Answer from the drawing. Dimensions are ordinates in mm from the lowest x, y and z of the part. A direction names the side the tool comes from. Give positions to 0.01 mm unless a question says otherwise; leave off trailing zeros. Loops run counter-clockwise (first coordinate to the right, second up) from the corner with the lowest first, then second, coordinate; pieces in that order, holes last.
Item 1: Consider line 1 along X through (y, z) = (3.35, 15.5); line 2 along Y through (x, z) = (4, 23.15); line 3 along X through (y, z) = (2.3, 5.5). Determine where each line is inside the solid, lowest interval first.
Item 2: Each of these flat-tipped pins is pushed along its axis until it touches: pin 1 Ø3 at (x, y) = (29, 2) entering from -Z; pin 2 Ø1.8 at (x, y) = (37.5, 3) entering from -Z; pin 3 Ø2 at (y, z) = (4, 9) entering from +X. Where does it stop, or does it pass through?
Item 3: Section C-C, the plane x = 20 is taken. Give the vertices of the cut face in (y, z), and give its area (3 significant figures).
Item 4: Section A-A, the plane x = 36 is taken. Give the vertices of the cut face in (y, z), and give its area (3 significant figures).
Item 5: Section D-D, the plane z = 2 is taken. Give the vertices of the cut face in (x, y).
Item 6: Section B-B, the plane y = 3.95 is taken. Give the vertices of the cut face in (x, z).
Item 7: The mould has two halves that part along X. Classify the marked faces 1, 2, 3 and 4: pulls with the +X half, pulls with the -X half, needs draft (parallel to the pull), parting line crosses it, or undercut.
Item 8: A tool of negligible diameter and unlimited length cuts with its end or side. For the marked faces 5, 6 and 7, from which of +Z, -Z, +X, -X, +Y, -Y can it reach the whole face along a straight path? Write none if from no direction.
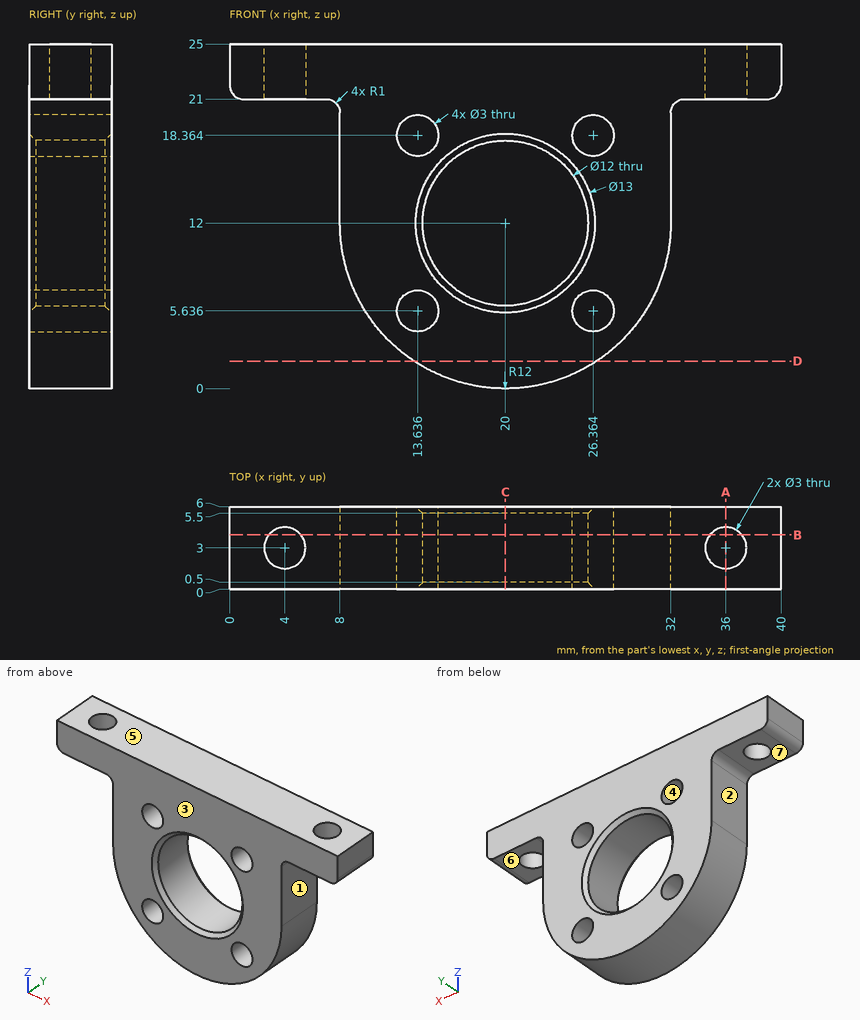
Worked answers:
1. line 1: x = 8 to 15.13, 24.87 to 32
1. line 2: y = 0 to 1.5, 4.5 to 6
1. line 3: x = 9.91 to 12.14, 15.13 to 24.87, 27.86 to 30.09
2. pin 1: stops at z = 2.63
2. pin 2: stops at z = 21
2. pin 3: stops at x = 31.83
3. outline: (0, 0) - (6, 0) - (6, 5.5) - (5.5, 6) - (0.5, 6) - (0, 5.5) - close; (0, 18.5) - (0.5, 18) - (5.5, 18) - (6, 18.5) - (6, 25) - (0, 25) - close
3. area: 77.5 mm2
4. outline: (0, 21) - (1.5, 21) - (1.5, 25) - (0, 25) - close; (4.5, 21) - (6, 21) - (6, 25) - (4.5, 25) - close
4. area: 12.0 mm2
5. outline: (13.37, 0) - (26.63, 0) - (26.63, 6) - (13.37, 6) - close
6. outline: (0, 22) arc R1 ccw to (1, 21) - (2.84, 21) - (2.84, 25) - (0, 25) - close; (5.16, 21) - (7, 21) arc R1 cw to (8, 20) - (8, 12) arc R12 ccw to (32, 12) - (32, 20) arc R1 cw to (33, 21) - (34.84, 21) - (34.84, 25) - (5.16, 25) - close; (37.16, 21) - (39, 21) arc R1 ccw to (40, 22) - (40, 25) - (37.16, 25) - close; hole circle Ø3 at (13.64, 5.64); hole circle Ø3 at (13.64, 18.36); hole circle Ø12 at (20, 12); hole circle Ø3 at (26.36, 5.64); hole circle Ø3 at (26.36, 18.36)
7. face 1: pulls with the +X half
7. face 2: pulls with the -X half
7. face 3: needs draft
7. face 4: undercut
8. face 5: +Z, +X, -X, +Y, -Y
8. face 6: -Z, +X, +Y, -Y
8. face 7: -Z, -X, +Y, -Y
